Autodesk Inventor part; units mm, degrees
ref_plane "YZ Plane" through (0, 0, 0) normal (1, 0, 0) x (0, 1, 0)
ref_plane "XZ Plane" through (0, 0, 0) normal (0, 1, 0) x (-1, 0, 0)
ref_plane "XY Plane" through (0, 0, 0) normal (0, 0, 1) x (1, 0, 0)
sketch "Sketch1" plane through (0, 0, 0) normal (0, 1, 0) x (-1, 0, 0)
  line L0 (0, 0) -> (0, -110) construction
  line L1 (4, 0) -> (4, -110)
  line L2 (-4, -110) -> (-4, 0)
  arc A0 (4, 0) -> (-4, 0) centre (0, 0) ccw
  arc A1 (-4, -110) -> (4, -110) centre (0, -110) ccw
  circle A2 centre (0, 0) radius 2.1
  circle A3 centre (0, -110) radius 2.1
  circle A4 centre (7, -80) radius 2.1
  circle A5 centre (7, -80) radius 5
  point P0 (0, -55)
  point P1 (4, -76)
  point P2 (4, -84)
  dimension "d0" = 110
  dimension "d1" = 8
  dimension "d2" = 4.2
  dimension "d3" = 4.2
  dimension "d6" = 4.2
  dimension "d9" = 80
  dimension "d10" = 3
  dimension "d11" = 10
extrude "Extrusion1" add sketch "Sketch1" along normal blind 5
Model file for the job. Use its own axes, mm. Give positions to 0.01 mm unless a question says otherwise; leave off trailing zeros. Write each loop counter-clockwise with the first axis right and the second up, starting at its lowest first coordinate (ties: lowest second). Pieces come first, ordered by that corner, then holes. Notation, with made-up numbers: M 19.5,59.25 L 53.5,59.25 A9 cw 53.5,63.25 Z; hole C 32,65 d9. An arc over 180 degrees is marked long. One line per item, written item: value. Start each with the question number.
Q1. Saw through at A-A, the plane x = 0. Write the cut outline in (y, z).
Q2. Drop flat-ended pins along their axis: pin 1 Ø4 at (x, z) = (-6.5, -23.5) entering from +Y; pin 2 Ø1.5 at (x, y) = (-9, 1) entering from -Z; pin 3 Ø1.5 at (y, z) = (2, -35) entering from -X. Give the stop position or say it passes through.
Q3. Probe probe 1 along Z at (x, y) = (0, 3.4); probe 2 along Z at (x, y) = (-7, 3.15); probe 3 along X at (y, z) = (2.95, -87). List the from-to ranges inside material, lowest first. Write a range as [from, to].
Q4. Two-plate mould, pull along Z, no slides. Class faces 1 (the flat face through (-4, 2, -97)), 2 (the cylindrical face through (-2.003, 2.465, -0.631)), 3 (the cylindrical face through (0.46, 2.46, -107.95)), 4 (the cylindrical face through (0, 2, 4)): +Z half, -Z half, draft (parallel to the pull), parting line (faces both ways), or undercut.
Q5. Saw through at C-C, the plane z = -80. Write the cut outline in (x, y).
Q6. Saw through at D-D, the plane x = -7. Write the cut outline in (y, z), plus the area to 3 significant figures.
Q7. Saw through at B-B, the plane y = 0.75. Write the cut outline in (x, z).
Output values:
1. outline: M 0,-114 L 5,-114 L 5,-112.1 L 0,-112.1 Z; M 0,-107.9 L 5,-107.9 L 5,-2.1 L 0,-2.1 Z; M 0,2.1 L 5,2.1 L 5,4 L 0,4 Z
2. pin 1: passes through
2. pin 2: stops at z = -84.84
2. pin 3: stops at x = -4
3. probe 1: z = [-114, -112.1], [-107.9, -2.1], [2.1, 4]
3. probe 2: z = [-85, -82.1], [-77.9, -75]
3. probe 3: x = [-4, 4]
4. face 1: draft
4. face 2: undercut
4. face 3: undercut
4. face 4: +Z half
5. outline: M -12,0 L -9.1,0 L -9.1,5 L -12,5 Z; M -4.9,0 L 4,0 L 4,5 L -4.9,5 Z
6. outline: M 0,-85 L 5,-85 L 5,-82.1 L 0,-82.1 Z; M 0,-77.9 L 5,-77.9 L 5,-75 L 0,-75 Z
6. area: 29.0 mm²
7. outline: M -4,-110 A4 ccw 4,-110 L 4,0 A4 ccw -4,0 L -4,-76 A5 ccw long -4,-84 Z; hole C -7,-80 d4.2; hole C 0,-110 d4.2; hole C 0,0 d4.2
